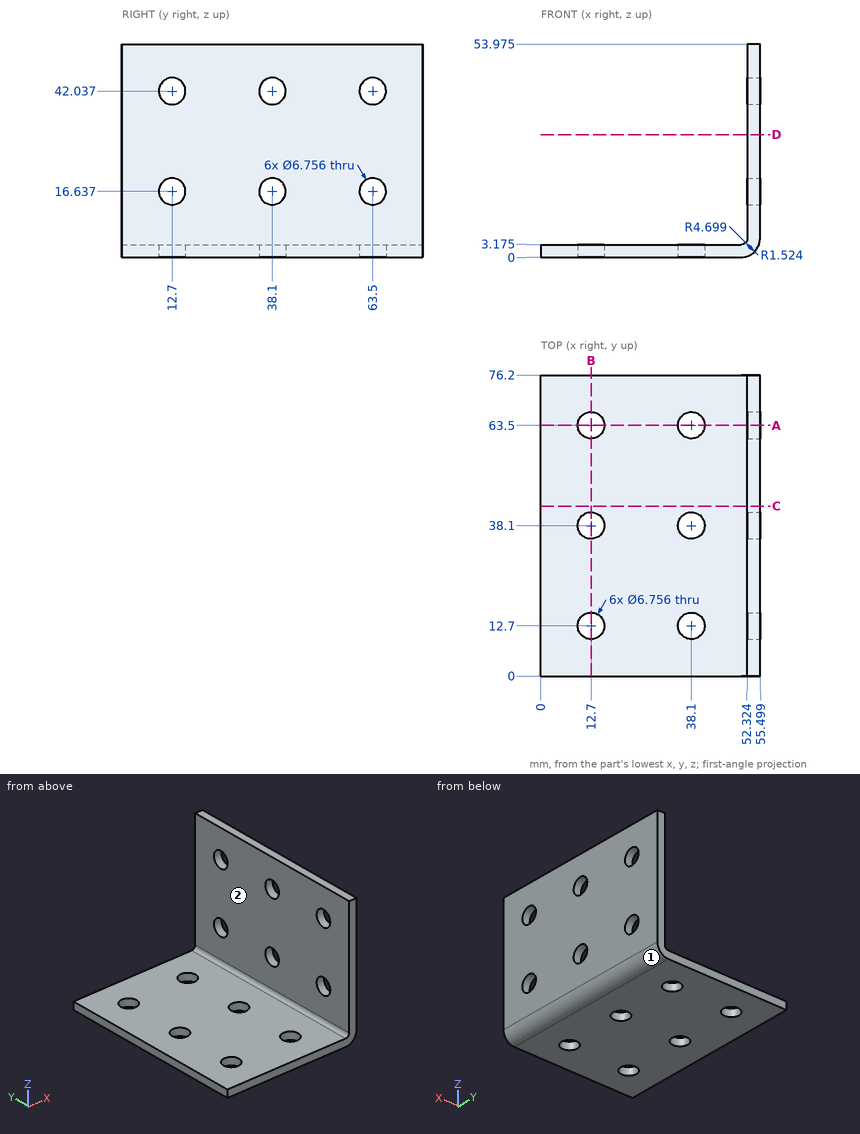
Answer from the drawing. Dimensions are ordinates in mm from the lowest x, y and z of the part. A direction names the side the tool comes from. Give positions to 0.01 mm unless a question says otherwise; leave off trailing zeros. Write each loop counter-clockwise with the first axis right and the second up, starting at its lowest first coordinate (ties: lowest second). Pieces come first, ordered by that corner, then holes. Notation, with made-up numbers: (-23, 17) - (25, 17) arc R25 cw to (25, 29) - close; hole circle Ø2 at (56, 28). An arc over 180 degrees is marked (long way). Answer in a Markdown table with one row per item. Add a question column.
Item 1: Section C-C, the plane y = 43 is taken. Write down the section's boundary in (x, z) (1 decimal).
Item 2: Section D-D, the plane z = 31 is taken. Write down the section's boundary in (x, y).
Item 3: Section A-A, the plane y = 63.5 is taken. Write down the section's boundary in (x, z) (1 decimal).
Item 4: Flat-ended cylindrical pins translate along their axes: P1, Ø8, axis at x = 12.7, y = 12.7, coming from the +Z side (3 decimals); P2, Ø6, axis at x = 38.1, y = 12.7, coming from the +Z side; P3, Ø24.5, axis at y = 38.5, z = 22, coming from the -X side. Find the tip coordinate at first contact, or state that the pin passes through.
Item 5: Find the intervals of material crossed by L1, parallel to Y at x = 38.1, z = 0.7; L2, parallel to Y at x = 12, z = 1 (1 decimal); L3, parallel to X at y = 38, z = 1 (1 decimal), in increasing order.
Item 6: A tool of negligible diameter and unlimited length cuts with its end or side. For the marked faces 1 and 2, from which of +Z, -Z, +X, -X, +Y, -Y can it reach the whole face along a straight path? Write none if from no direction.
Item 7: Section B-B, the plane x = 12.7 is taken. Write down the section's boundary in (y, z) (1 decimal).
Recorded:
| question | item | result |
|---|---|---|
| 1 | outline | (0, 0) - (50.8, 0) arc R4.7 ccw to (55.5, 4.7) - (55.5, 54) - (52.3, 54) - (52.3, 4.7) arc R1.5 cw to (50.8, 3.2) - (0, 3.2) - close |
| 2 | outline | (52.32, 0) - (55.5, 0) - (55.5, 76.2) - (52.32, 76.2) - close |
| 3 | outline | (0, 0) - (9.3, 0) - (9.3, 3.2) - (0, 3.2) - close; (16.1, 0) - (34.7, 0) - (34.7, 3.2) - (16.1, 3.2) - close; (41.5, 0) - (50.8, 0) arc R4.7 ccw to (55.5, 4.7) - (55.5, 13.3) - (52.3, 13.3) - (52.3, 4.7) arc R1.5 cw to (50.8, 3.2) - (41.5, 3.2) - close; (52.3, 20) - (55.5, 20) - (55.5, 38.7) - (52.3, 38.7) - close; (52.3, 45.4) - (55.5, 45.4) - (55.5, 54) - (52.3, 54) - close |
| 4 | P1 | stops at z = 3.175 |
| 4 | P2 | passes through |
| 4 | P3 | stops at x = 52.32 |
| 5 | L1 | y = 0 to 9.32, 16.08 to 34.72, 41.48 to 60.12, 66.88 to 76.2 |
| 5 | L2 | y = 0 to 9.4, 16 to 34.8, 41.4 to 60.2, 66.8 to 76.2 |
| 5 | L3 | x = 0 to 9.3, 16.1 to 34.7, 41.5 to 53.7 |
| 6 | face 1 | -Z, +X, +Y, -Y |
| 6 | face 2 | +Z, -X, +Y, -Y |
| 7 | outline | (0, 0) - (9.3, 0) - (9.3, 3.2) - (0, 3.2) - close; (16.1, 0) - (34.7, 0) - (34.7, 3.2) - (16.1, 3.2) - close; (41.5, 0) - (60.1, 0) - (60.1, 3.2) - (41.5, 3.2) - close; (66.9, 0) - (76.2, 0) - (76.2, 3.2) - (66.9, 3.2) - close |
